Autodesk Inventor part; units mm, degrees
ref_plane "YZ Plane" through (0, 0, 0) normal (1, 0, 0) x (0, 1, 0)
ref_plane "XZ Plane" through (0, 0, 0) normal (0, 1, 0) x (-1, 0, 0)
ref_plane "XY Plane" through (0, 0, 0) normal (0, 0, 1) x (1, 0, 0)
sketch "Sketch1" plane through (0, 0, 0) normal (0, 0, 1) x (1, 0, 0)
  line L0 (1.27, -1.27) -> (-1.27, -1.27)
  line L1 (-1.27, -1.27) -> (-1.27, 1.27)
  line L2 (-1.27, 1.27) -> (1.27, 1.27)
  line L3 (1.27, 1.27) -> (1.27, -1.27)
  line L4 (1.27, -1.27) -> (-1.27, 1.27) construction
  line L5 (-1.27, -1.27) -> (1.27, 1.27) construction
  point P0 (0, 0)
  dimension "d0" = 2.54
  dimension "d1" = 2.54
extrude "Extrusion1" add sketch "Sketch1" along normal blind 8.382
sketch "Sketch2" plane through (0, 0, 8.382) normal (0, 0, 1) x (1, 0, 0)
  line L0 (0.5715, 0.5715) -> (-0.5715, 0.5715)
  line L1 (-0.5715, 0.5715) -> (-0.5715, -0.5715)
  line L2 (-0.5715, -0.5715) -> (0.5715, -0.5715)
  line L3 (0.5715, -0.5715) -> (0.5715, 0.5715)
  line L4 (0.5715, 0.5715) -> (-0.5715, -0.5715) construction
  line L5 (-0.5715, 0.5715) -> (0.5715, -0.5715) construction
  point P0 (0, 0)
  dimension "d4" = 1.143
extrude "Extrusion2" cut sketch "Sketch2" against normal blind 6.35
chamfer "Chamfer1" distance 0.381 angle 45 4 edges at (0, 0.5715, 8.382) (-0.5715, 0, 8.382) (0, -0.5715, 8.382) (0.5715, 0, 8.382)
sketch "Sketch3" plane through (0, 0, 0) normal (0, 0, -1) x (-1, 0, 0)
  line L0 (0.4445, -0.4445) -> (-0.4445, -0.4445)
  line L1 (-0.4445, -0.4445) -> (-0.4445, 0.4445)
  line L2 (-0.4445, 0.4445) -> (0.4445, 0.4445)
  line L3 (0.4445, 0.4445) -> (0.4445, -0.4445)
  line L4 (0.4445, -0.4445) -> (-0.4445, 0.4445) construction
  line L5 (-0.4445, -0.4445) -> (0.4445, 0.4445) construction
  point P0 (0, 0)
  dimension "d10" = 0.889
extrude "Extrusion3" add sketch "Sketch3" along normal blind 3.302
chamfer "Chamfer2" distance 0.381 angle 45 4 edges at (0, 0.4445, -3.302) (-0.4445, 0, -3.302) (0, -0.4445, -3.302) (0.4445, 0, -3.302)
pattern_linear "Rectangular Pattern1" count 2 spacing 2.54 along (1, 0, 0) of "Extrusion1", "Extrusion2", "Chamfer1", "Extrusion3", "Chamfer2"
equation "\"d1\" = d0"
properties part number "2  female pin"
The listing builds one solid part. Answer for the finished solid, in the listing's coordinates (mm). A direction names the side the tool comes from. Give positions to 0.01 mm unless a question says otherwise; leave off trailing zeros. Write each loop counter-clockwise with the first axis right and the second up, starting at its lowest first coordinate (ties: lowest second). Pieces come first, ordered by that corner, then holes. Notation, with made-up numbers: M -40,84 L -23,84 A19 cw -23,91 Z; hole C -21,3.25 d11. An arc over 180 degrees is marked long. Write each question's results on one line, items separated by ' | '.
Q1. Consider L1, parallel to X at y = -0.45, z = 7.25; L2, parallel to Y at x = -0.15, z = 4; L3, parallel to Z at x = 1.9, y = -1.05. Determine where each line is inside the solid, lowest interval first. Write a range as from..to.
Output values:
L1: -1.27..-0.57, 0.57..1.97, 3.11..3.81 | L2: -1.27..-0.57, 0.57..1.27 | L3: 0..8.38
Q2. Section C-C, the plane y = -0.7 is taken. Write down the section's boundary in (x, z).
Output values:
outline: M -1.27,0 L 3.81,0 L 3.81,8.38 L 3.49,8.38 L 3.24,8.13 L 1.84,8.13 L 1.59,8.38 L 0.95,8.38 L 0.7,8.13 L -0.7,8.13 L -0.95,8.38 L -1.27,8.38 Z
Q3. Section A-A, the plane z = 3.5 is taken. Write down the section's boundary in (x, y).
Output values:
outline: M -1.27,-1.27 L 3.81,-1.27 L 3.81,1.27 L -1.27,1.27 Z; hole M -0.57,-0.57 L 0.57,-0.57 L 0.57,0.57 L -0.57,0.57 Z; hole M 1.97,-0.57 L 3.11,-0.57 L 3.11,0.57 L 1.97,0.57 Z
Q4. For a pull along X with two mould halves and no side action, classify faces 1 (the flat face through (0, 0.572, 5)), 2 (the flat face through (-1.27, 0, 4)), 3 (the flat face through (2.5, 0.444, -1.4)) as released by +X, released by -X, zero draft, split by the parting line, or undercut.
Output values:
face 1: undercut | face 2: released by -X | face 3: zero draft
Q5. Flat-ended cylindrical pins translate along their axes: P1, Ø1.3, axis at x = 1, y = 0.5, coming from the -Z side; P2, Ø1, axis at x = 3, y = 1, coming from the -Z side; P3, Ø1.5, axis at y = -1, z = -1.5, coming from the -X side. Find the tip coordinate at first contact, or state that the pin passes through.
Output values:
P1: z = -3 | P2: z = 0 | P3: x = -0.44
Q6. Section B-B, the plane z = -1 is taken. Write down the section's boundary in (x, y).
Output values:
outline: M -0.44,-0.44 L 0.44,-0.44 L 0.44,0.44 L -0.44,0.44 Z; M 2.1,-0.44 L 2.98,-0.44 L 2.98,0.44 L 2.1,0.44 Z
Q7. Section D-D, the plane x = -0.2 is taken. Write down the section's boundary in (y, z).
Output values:
outline: M -1.27,0 L -0.44,0 L -0.44,-2.92 L -0.2,-3.17 L 0.2,-3.17 L 0.44,-2.92 L 0.44,0 L 1.27,0 L 1.27,8.38 L 0.95,8.38 L 0.57,8 L 0.57,2.03 L -0.57,2.03 L -0.57,8 L -0.95,8.38 L -1.27,8.38 Z
Q8. A tool of negligible diameter and unlimited length cuts with its end or side. For faces 4 (the flat face through (0, 0.444, -1)), 5 (the flat face through (2.984, 0, -1)), 6 (the flat face through (-0.444, 0, -1)), from which of +Z, -Z, +X, -X, +Y, -Y can it reach the whole face along a straight path? Write none if from no direction.
Output values:
face 4: -Z, +X, -X, +Y | face 5: -Z, +X, +Y, -Y | face 6: -Z, -X, +Y, -Y
